from build123d import *

# Parameters (mm, degrees)
SKETCH_1_R          = 8
EXTRUDE_1_DEPTH     = 32
SKETCH_2_R          = 9
EXTRUDE_2_DEPTH     = 22
CUT_EXTRUDE_1_REACH = 36.438
SKETCH_3_R          = 3


with BuildPart() as part:
    # 草图1 → 凸台-拉伸1 (new body)
    with BuildSketch(Plane.XY):
        Circle(SKETCH_1_R)
    extrude(amount=EXTRUDE_1_DEPTH)

    # 草图2 → 凸台-拉伸2 (add)
    with BuildSketch(Plane(origin=(0, 0, 0), x_dir=(-1, 0, 0), z_dir=(0, 0, -1))):
        Circle(SKETCH_2_R)
    extrude(amount=-EXTRUDE_2_DEPTH)

    # 草图3 → 切除-拉伸1 (cut, up to next)
    with BuildSketch(Plane.XY.offset(32), mode=Mode.PRIVATE) as cut_extrude_1_sk1:
        Circle(SKETCH_3_R)
    cut_extrude_1_tool1 = extrude(cut_extrude_1_sk1.sketch, amount=-CUT_EXTRUDE_1_REACH, mode=Mode.PRIVATE) & part.part
    add(cut_extrude_1_tool1.solids().sort_by_distance((0, 0, 32))[0], mode=Mode.SUBTRACT)


solid = part.part
Read the model definition and answer for the solid it produces. Units are mm, in the model's axes. A direction names the side the tool comes from. Coordinates: 2 decimals unless noted, no trailing zeros. Loops run counter-clockwise (first coordinate to the right, second up) from the corner with the lowest first, then second, coordinate; pieces in that order, holes last. Notation, with made-up numbers: (37, 79.25) -> (89, 79.25) arc R8 ccw to (89, 93.25) -> close; hole circle Ø11 at (-35, 1). An arc over 180 degrees is marked (long way). Answer in a Markdown table with one row per item.
Item 1: Each of these flat-tipped pins is pushed along its axis until it touches: P1, Ø3, axis at x = 5.5, z = 21.5, coming from the +Y side; P2, Ø4, axis at y = -4, z = 7.5, coming from the +X side. Where does it stop, or does it pass through?
Returned:
| item | result |
|---|---|
| P1 | stops at y = 8.06 |
| P2 | stops at x = 8.77 |
Item 2: A cutting plane is placed at A-A on x = 0. Determine the outline of the cut face in (y, z), plus the area to 3 significant figures.
Returned:
| item | result |
|---|---|
| outline | (-9, 0) -> (-3, 0) -> (-3, 32) -> (-8, 32) -> (-8, 22) -> (-9, 22) -> close; (3, 0) -> (9, 0) -> (9, 22) -> (8, 22) -> (8, 32) -> (3, 32) -> close |
| area | 364 mm^2 |
Item 3: A cutting plane is placed at C-C on z = 6. Determine the outline of the cut face in (x, y).
Returned:
| item | result |
|---|---|
| outline | circle Ø18 at (0, 0); hole circle Ø6 at (0, 0) |
Item 4: For faces 1 (the cylindrical face through (-1.73, -7.81, 26.93)), 2 (the flat face through (0, -4, 0)), determine the directions among +Z, -Z, +X, -X, +Y, -Y from which every point of the face is accessible in a straight line to the end or side of a thin tool.
Returned:
| item | result |
|---|---|
| face 1 | +Z |
| face 2 | -Z, +X, -X, +Y, -Y |
Item 5: Straight lines are drawn through the part: line 1 along Y through (x, z) = (0, 15); line 2 along Z through (x, y) = (-7.5, 3.5); line 3 along Y through (x, z) = (0, 24.5). For each, find the intervals that lie inside material, in ascending order. Write a range as [from, to].
Returned:
| item | result |
|---|---|
| line 1 | y = [-9, -3], [3, 9] |
| line 2 | z = [0, 22] |
| line 3 | y = [-8, -3], [3, 8] |
Item 6: A cutting plane is placed at D-D on x = -6.5. Determine the outline of the cut face in (y, z), plus the area to 3 significant figures.
Returned:
| item | result |
|---|---|
| outline | (-6.22, 0) -> (6.22, 0) -> (6.22, 22) -> (4.66, 22) -> (4.66, 32) -> (-4.66, 32) -> (-4.66, 22) -> (-6.22, 22) -> close |
| area | 367 mm^2 |
